For this review, take the finished solid that the model builds, in its own axes (mm). Round coordinates to 2 decimals unless told otherwise and drop trailing zeros. Loops run counter-clockwise (first coordinate to the right, second up) from the corner with the lowest first, then second, coordinate; pieces in that order, holes last.
1. To check wall thickness, follow line 1 along Y through (x, z) = (47, 2.3); line 2 along Y through (x, z) = (38.5, 2.2); line 3 along X through (y, z) = (76, 2.5). State the ranges of each line that lie inside material, in increasing order.
2. Consider section B-B on y = 58.5. State the section outline as (x, z) points.
3. Draft analysis for pull direction Y (two halves, no side actions). For faces 1 (the cylindrical face through (-2.75, -12.4, 1.52)), 2 (the cylindrical face through (19.949, 32.646, 1.52)), 3 (the flat face through (16, -2, 0)), state which applies: released by +Y, released by -Y, zero draft, split by the parting line, or undercut.
4. Clearance check with flat-ended pins moving along their axes: pin 1 Ø1 at (y, z) = (-108, 2.5) entering from -X; pin 2 Ø0.9 at (y, z) = (12, 2) entering from -X. State where each tip first meets the part, or that it passes through.
5. Consider section A-A on x = 0. State how many separate pieces and enclosed holes the cut face has, then the cut area to 3 significant figures.
from build123d import *

# Parameters (mm, degrees)
F1_DEPTH = 2.9972
F2_R     = 2.54
F2_R_2   = 12.7
F3_DEPTH = 2.9982001
F4_R     = 3.175
F5_DEPTH = 2.9982001


# Not quite as in the source:
# - a feature names something its author has since deleted; it is built from what else it names


with BuildPart() as f1:
    # F0 (on Top) → F1 (new body)
    with BuildSketch(Plane.XY):
        with BuildLine():
            Line((-50.8, 69.1337430724), (-50.8, 0))
            ThreePointArc((-50.8, 0), (0, -50.8), (50.8, 0))
            Line((50.8, 0), (50.8, 68.084156834))
            ThreePointArc((50.8, 68.084156834), (51.3066265414, 76.856454963), (52.8197694085, 85.5121053476))
            add(Edge.make_bspline(
                [(-52.4169124656, 84.7479370585), (-59.7763542356, 119.901201468), (-79.0847149078, 143.3209937269), (-48.7989520232, 156.4254085379), (48.9543407971, 156.6289051226), (78.6905979985, 142.9845070095), (61.240777086, 121.355239199), (52.8197694085, 85.5121053476)],
                knots=[0.016652167, 0.016652167, 0.016652167, 0.016652167, 0.2315423779, 0.3598652356, 0.6401347644, 0.7684576221, 0.9823940037, 0.9823940037, 0.9823940037, 0.9823940037], degree=3))
            ThreePointArc((-52.4169124656, 84.7479370585), (-51.205306023, 76.982587888), (-50.8, 69.1337430724))
        make_face()
        with BuildLine():
            ThreePointArc((-40.8635060245, 77.3464568111), (-46.0941000823, 74.9267134219), (-44.5517945725, 80.47969154))
            ThreePointArc((-44.5517945725, 80.47969154), (-41.9829119668, 79.7662002004), (-40.8635060245, 77.3464568111))
        make_face(mode=Mode.SUBTRACT)
        with BuildLine():
            ThreePointArc((-44.8219086152, 95.9806605486), (-45.4423549678, 94.0952214319), (-47.0612035208, 92.9466729124))
            ThreePointArc((-47.0612035208, 92.9466729124), (-51.0712627717, 95.1875833011), (-48.645629391, 99.0886802324))
            ThreePointArc((-48.645629391, 99.0886802324), (-45.9942932581, 98.444429355), (-44.8219086152, 95.9806605486))
        make_face(mode=Mode.SUBTRACT)
        with BuildLine():
            ThreePointArc((-50.4062777497, 114.1937690523), (-50.9612142113, 112.4004782074), (-52.4320365242, 111.2340613632))
            ThreePointArc((-52.4320365242, 111.2340613632), (-56.5676237816, 113.1156399423), (-54.5876780098, 117.2050451135))
            ThreePointArc((-54.5876780098, 117.2050451135), (-51.7258392336, 116.7701954365), (-50.4062777497, 114.1937690523))
        make_face(mode=Mode.SUBTRACT)
        with BuildLine():
            ThreePointArc((-57.3376559554, 131.938021535), (-57.88209946, 130.1601583445), (-59.3287095139, 128.9920249594))
            ThreePointArc((-59.3287095139, 128.9920249594), (-63.4641851685, 130.7679359381), (-61.6688548547, 134.8950181711))
            ThreePointArc((-61.6688548547, 134.8950181711), (-58.7224473789, 134.5601920582), (-57.3376559554, 131.938021535))
        make_face(mode=Mode.SUBTRACT)
        with BuildLine():
            ThreePointArc((-53.7960603193, 144.1342135781), (-56.4975490613, 140.9947212483), (-60.0048238397, 143.1977821056))
            ThreePointArc((-60.0048238397, 143.1977821056), (-57.8198491671, 147.1936551107), (-53.8884721201, 144.8946575233))
            ThreePointArc((-53.8884721201, 144.8946575233), (-53.8192479413, 144.5172328122), (-53.7960603193, 144.1342135781))
        make_face(mode=Mode.SUBTRACT)
        with BuildLine():
            ThreePointArc((-34.9702627037, 147.0482904702), (-37.995578786, 143.8768208227), (-41.3061491445, 146.7492555085))
            ThreePointArc((-41.3061491445, 146.7492555085), (-38.4509946725, 150.2085361827), (-34.9856719085, 147.3607180735))
            ThreePointArc((-34.9856719085, 147.3607180735), (-34.9741173448, 147.2046941553), (-34.9702627037, 147.0482904702))
        make_face(mode=Mode.SUBTRACT)
        with BuildLine():
            ThreePointArc((-15.9590420103, 148.2631928317), (-19.0948463149, 145.0884347783), (-22.3080742607, 148.1848074146))
            ThreePointArc((-22.3080742607, 148.1848074146), (-19.2571889586, 151.4358037169), (-15.9634837046, 148.4310768101))
            ThreePointArc((-15.9634837046, 148.4310768101), (-15.9601526281, 148.3471641942), (-15.9590420103, 148.2631928317))
        make_face(mode=Mode.SUBTRACT)
        with BuildLine():
            ThreePointArc((47.2575965607, 77.582145781), (41.6326151645, 75.5626864082), (44.6886415002, 80.6987680763))
            ThreePointArc((44.6886415002, 80.6987680763), (46.5325779568, 79.6016051539), (47.2575965607, 77.582145781))
        make_face(mode=Mode.SUBTRACT)
        with BuildLine():
            ThreePointArc((47.4797824009, 93.1003405079), (45.3705359663, 96.9606098577), (49.1428743284, 99.2233655354))
            ThreePointArc((49.1428743284, 99.2233655354), (50.9174308294, 98.1072314537), (51.6095262724, 96.1283908938))
            ThreePointArc((51.6095262724, 96.1283908938), (50.3119331553, 93.5679283583), (47.4797824009, 93.1003405079))
        make_face(mode=Mode.SUBTRACT)
        with BuildLine():
            ThreePointArc((3.0909579897, 148.6372462056), (-0.1029362656, 145.4623024254), (-3.2588171329, 148.675034047))
            ThreePointArc((-3.2588171329, 148.675034047), (-0.0872347979, 151.8122446002), (3.0906506924, 148.6814190904))
            ThreePointArc((3.0906506924, 148.6814190904), (3.0908811644, 148.6593331824), (3.0909579897, 148.6372462056))
        make_face(mode=Mode.SUBTRACT)
        with BuildLine():
            ThreePointArc((22.137110859, 148.2255283412), (18.8449293043, 145.1249914855), (15.7921571233, 148.4615121573))
            ThreePointArc((15.7921571233, 148.4615121573), (19.044817873, 151.4717417271), (22.1379334659, 148.2977978171))
            ThreePointArc((22.1379334659, 148.2977978171), (22.1377278075, 148.2616607384), (22.137110859, 148.2255283412))
        make_face(mode=Mode.SUBTRACT)
        with BuildLine():
            ThreePointArc((41.1358520444, 146.797176727), (37.6674396013, 143.9372524612), (34.8157468695, 147.4124359448))
            ThreePointArc((34.8157468695, 147.4124359448), (38.132825935, 150.2683923102), (41.1500700749, 147.0973139308))
            ThreePointArc((41.1500700749, 147.0973139308), (41.1465135754, 146.9470770399), (41.1358520444, 146.797176727))
        make_face(mode=Mode.SUBTRACT)
        with BuildLine():
            ThreePointArc((52.9867605228, 111.3442691981), (51.1303654682, 115.3814686532), (55.1283946905, 117.3207840933))
            ThreePointArc((55.1283946905, 117.3207840933), (56.6965282926, 116.1646916046), (57.294259448, 114.3104234734))
            ThreePointArc((57.294259448, 114.3104234734), (55.9199455551, 111.6954369449), (52.9867605228, 111.3442691981))
        make_face(mode=Mode.SUBTRACT)
        with BuildLine():
            ThreePointArc((59.8190768743, 143.166925299), (55.922941879, 141.0690853743), (53.7138004196, 144.9032077333))
            ThreePointArc((53.7138004196, 144.9032077333), (57.1845775976, 147.2735561917), (59.9664431146, 144.1229895318))
            ThreePointArc((59.9664431146, 144.1229895318), (59.9293852896, 143.6393120499), (59.8190768743, 143.166925299))
        make_face(mode=Mode.SUBTRACT)
        with BuildLine():
            ThreePointArc((59.7670804201, 129.1468155623), (57.9403922201, 133.2339684449), (62.0166331459, 135.0848785944))
            ThreePointArc((62.0166331459, 135.0848785944), (63.5167589772, 133.9209947171), (64.0844760149, 132.109172277))
            ThreePointArc((64.0844760149, 132.109172277), (62.7057943311, 129.4911834484), (59.7670804201, 129.1468155623))
        make_face(mode=Mode.SUBTRACT)
    extrude(amount=F1_DEPTH)

    # F2 (on face) → F3 (cut, through all)
    with BuildSketch(Plane.XY.offset(2.9972)):
        with Locations((23.8125, 0)):
            Circle(F2_R)
        with Locations((11.90625, 20.6222299276)):
            Circle(F2_R)
        with Locations((-23.8125, 0)):
            Circle(F2_R)
        with Locations((-11.90625, -20.6222299276)):
            Circle(F2_R)
        with Locations((11.90625, -20.6222299276)):
            Circle(F2_R)
        with Locations((-11.90625, 20.6222299276)):
            Circle(F2_R)
        Circle(F2_R_2)
    extrude(amount=-F3_DEPTH, mode=Mode.SUBTRACT)

    # F4 (on face) → F5 (cut, through all)
    with BuildSketch(Plane.XY.offset(2.9972)):
        with Locations((-20.6375, 35.7451985412)):
            Circle(F4_R)
        with Locations((-41.275, 0)):
            Circle(F4_R)
        with Locations((-20.6375, -35.7451985412)):
            Circle(F4_R)
        with Locations((20.6375, -35.7451985412)):
            Circle(F4_R)
        with Locations((41.275, 0)):
            Circle(F4_R)
        with Locations((20.6375, 35.7451985412)):
            Circle(F4_R)
    extrude(amount=-F5_DEPTH, mode=Mode.SUBTRACT)

    # F6: F1 across plane


with BuildPart() as f1_1:
    add(f1.part)
    add(f1.part.mirror(Plane.XZ))


solid = f1_1.part
Resolved:
1. line 1: y = -152.97 to -98.96, -93.3 to -78.83, -76.33 to 76.33, 78.83 to 93.3, 98.96 to 152.97
1. line 2: y = -153.94 to -150.23, -143.97 to -1.54, 1.54 to 143.97, 150.23 to 153.94
1. line 3: x = -51.11 to -46.91, -41.16 to 41.33, 46.84 to 51.21
2. outline: (-50.8, 0) - (50.8, 0) - (50.8, 3) - (-50.8, 3) - close
3. face 1: undercut
3. face 2: undercut
3. face 3: zero draft
4. pin 1: stops at x = -58.87
4. pin 2: stops at x = -50.8
5. separate pieces: 4
5. enclosed holes: 0
5. area: 818 mm2
